```python
from build123d import *

# Parameters (mm, degrees)
BOSS_EXTRUDE1_DEPTH     = 70
CUT_EXTRUDE1_DEPTH      = 148.986485869
CUT_EXTRUDE1_DEPTH_BACK = 3
SKETCH3_R               = 4
CUT_EXTRUDE2_DEPTH      = 4
SKETCH4_R               = 2
CUT_EXTRUDE3_DEPTH      = 4


with BuildPart() as part:
    # Sketch1 → Boss-Extrude1 (new body)
    with BuildSketch(Plane(origin=(0, 0, 0), x_dir=(1, 0, 0), z_dir=(0, 1, 0))):
        Polygon((130, 10), (0, 10), (10, 0), (120, 0), align=None)
    extrude(amount=BOSS_EXTRUDE1_DEPTH)

    # Sketch2 → Cut-Extrude1 (cut, two sides: drawn at the far end of the back side and taken through both)
    with BuildSketch(Plane(origin=(0, 70, 0), x_dir=(1, 0, 0), z_dir=(0, 1, 0)).offset(-CUT_EXTRUDE1_DEPTH_BACK)):
        Polygon((125, 5), (5, 5), (10, 0), (120, 0), align=None)
    extrude(amount=CUT_EXTRUDE1_DEPTH + CUT_EXTRUDE1_DEPTH_BACK, mode=Mode.SUBTRACT)

    # Sketch3 → Cut-Extrude2 (cut)
    with BuildSketch(Plane.XY):
        with Locations((30, 5)):
            Circle(SKETCH3_R)
        with Locations((100, 5)):
            Circle(SKETCH3_R)
    extrude(amount=-CUT_EXTRUDE2_DEPTH, mode=Mode.SUBTRACT)

    # Sketch4 → Cut-Extrude3 (cut)
    with BuildSketch(Plane.XY):
        with Locations((30, 38.5)):
            Circle(SKETCH4_R)
        with Locations((100, 38.5)):
            Circle(SKETCH4_R)
    extrude(amount=-CUT_EXTRUDE3_DEPTH, mode=Mode.SUBTRACT)


solid = part.part
```
Geometry check sheet. Reference: the model listing, model coordinates, mm. A direction names the side the tool comes from. Give positions to 0.01 mm unless a question says otherwise; leave off trailing zeros. Loops run counter-clockwise (first coordinate to the right, second up) from the corner with the lowest first, then second, coordinate; pieces in that order, holes last. Notation, with made-up numbers: (54.25, -22) - (100.25, -22) arc R18 cw to (100.25, -7) - close; hole circle Ø9 at (78.5, 88.5). An arc over 180 degrees is marked (long way). Use CSV: the item, a comma, the result in double quotes. Start each with the question number.
Q1. Scan lines: probe 1 along Y at (x, z) = (30, -2.9); probe 2 along Y at (x, z) = (107.5, -3); probe 3 along X at (y, z) = (29, -4). Record each from-to range of solid material in increasing order. Write a range as from..to.
Q2. Section check D-D, the plane z = -7. Record the cut outline in (x, y), and give its area (3 significant figures).
Q3. Section check A-A, the plane z = -1.5. Record the cut outline in (x, y), and give its area (3 significant figures).
Q4. Access from +Z, -Z, +X, -X, +Y, -Y to the whole of each face (thin tool, end or side, straight path). Record for faces 4 (the face through (100, 5, -4)), 5 (the face through (66, 68, -5)), 6 (the face through (64, 33, 0)).
Q5. Section check B-B, the plane y = 5. Record the cut outline in (x, z).
Q6. Section check C-C, the plane x = 100. Record the cut outline in (y, z).
Q7. Release check for a two-part mould opening along Y. For faces 1 (the face through (64, 67, -3)), 2 (the face through (30, 39, -4)), 3 (the face through (125, 35, -5)) record: +Y half, -Y half, draft (parallel to the pull), parting line (faces both ways), or undercut.
Q8. Go/stop test with flat-tipped pins: pin 1 Ø4 at (y, z) = (57, -6) entering from +X; pin 2 Ø0.9 at (x, y) = (51, 69) entering from +Z; pin 3 Ø1.5 at (x, z) = (93.5, -3) entering from +Y. Record where each tip stops, or that it passes through.
Findings below:
1,probe 1,"y = 0..1, 9..36.5, 40.5..67"
1,probe 2,"y = 0..67"
1,probe 3,"x = 6..124"
2,outline,"(3, 0) - (127, 0) - (127, 70) - (3, 70) - close"
2,area,"8,680 mm^2"
3,outline,"(8.5, 0) - (121.5, 0) - (121.5, 67) - (8.5, 67) - close; hole circle Ø8 at (30, 5); hole circle Ø4 at (30, 38.5); hole circle Ø8 at (100, 5); hole circle Ø4 at (100, 38.5)"
3,area,"7,450 mm^2"
4,face 4,"+Z"
4,face 5,"+Z, +X, -X, +Y"
4,face 6,"+Z, +X, -X, +Y, -Y"
5,outline,"(0, -10) - (130, -10) - (120, 0) - (104, 0) - (104, -4) - (96, -4) - (96, 0) - (34, 0) - (34, -4) - (26, -4) - (26, 0) - (10, 0) - close"
6,outline,"(0, -10) - (70, -10) - (70, -5) - (67, -5) - (67, 0) - (40.5, 0) - (40.5, -4) - (36.5, -4) - (36.5, 0) - (9, 0) - (9, -4) - (1, -4) - (1, 0) - (0, 0) - close"
7,face 1,"+Y half"
7,face 2,"undercut"
7,face 3,"draft"
8,pin 1,"stops at x = 128"
8,pin 2,"stops at z = -5"
8,pin 3,"stops at y = 67"
